For this review, take the finished solid that the model builds, in its own axes (mm). Face numbers are marked on the shaded views. A direction names the side the tool comes from. Give positions to 0.01 mm unless a question says otherwise; leave off trailing zeros. Loops run counter-clockwise (first coordinate to the right, second up) from the corner with the lowest first, then second, coordinate; pieces in that order, holes last. Notation, with made-up numbers: (-13, -10) - (13, -10) arc R11 ccw to (13, 1) - close; hole circle Ø7 at (27, 43.5). An arc over 180 degrees is marked (long way). Put each result on its own line as item: value. Start each with the question number.
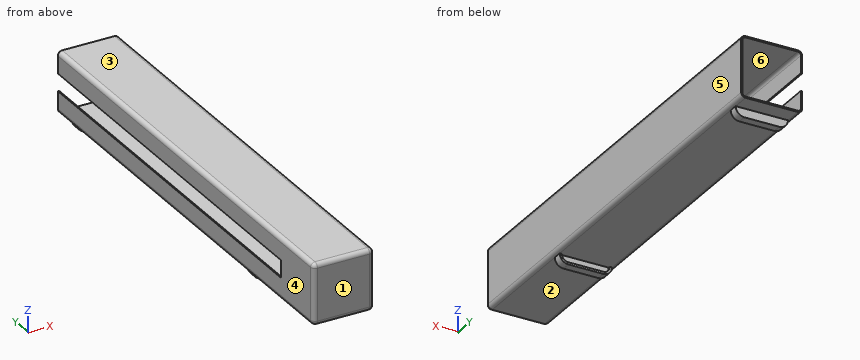
Autodesk Inventor part; units mm, degrees
ref_plane "YZ Plane" through (0, 0, 0) normal (1, 0, 0) x (0, 1, 0)
ref_plane "XY Plane" through (0, 0, 0) normal (0, 0, 1) x (1, 0, 0)
sketch "草图1" plane through (0, 0, 0) normal (0, 1, 0) x (-1, 0, 0)
  line L0 (0, 0) -> (-70, 0)
  line L1 (-70, 0) -> (-70, -70)
  line L2 (-70, -70) -> (0, -70)
  line L3 (0, -70) -> (0, 0)
  dimension "d0" = 70
  dimension "d1" = 70
extrude "拉伸1" add sketch "草图1" along normal blind 5
sketch "草图2" plane through (0, 5, 0) normal (0, 1, 0) x (1, 0, 0)
  line L0 (0, 70) -> (0, 0)
  line L1 (70, 70) -> (0, 70)
  line L2 (0, 0) -> (70, 0)
  line L3 (70, 0) -> (70, 70)
  line L4 (70, 70) -> (0, 70)
  line L5 (0, 70) -> (0, 0)
  line L6 (60, 60) -> (60, 10)
  line L7 (60, 10) -> (10, 10)
  line L8 (10, 10) -> (10, 60)
  line L9 (10, 60) -> (60, 60)
  dimension "d4" = 10
extrude "拉伸2" add sketch "草图2" along normal blind 60
fillet "圆角1" radius 5 8 edges at (0, 32.5, 0) (35, 0, 0) (0, 0, -35) (35, 0, -70) (70, 0, -35) (70, 32.5, -70) (70, 32.5, 0) (0, 32.5, -70)
sketch "草图3" plane through (0, 65, 0) normal (0, 1, 0) x (1, 0, 0)
  arc A0 (0, 5) -> (5, 0) centre (5, 5) ccw
  line L0 (5, 0) -> (65, 0)
  arc A1 (65, 0) -> (70, 5) centre (65, 5) ccw
  line L1 (70, 5) -> (70, 65)
  arc A2 (70, 65) -> (65, 70) centre (65, 65) ccw
  line L2 (65, 70) -> (5, 70)
  arc A3 (5, 70) -> (0, 65) centre (5, 65) ccw
  line L3 (0, 65) -> (0, 5)
  line L4 (60, 60) -> (60, 10)
  line L5 (60, 10) -> (10, 10)
  line L6 (10, 10) -> (10, 60)
  line L7 (10, 60) -> (60, 60)
  line L8 (68.5, 65) -> (68.5, 5)
  arc A4 (65, 1.5) -> (68.5, 5) centre (65, 5) ccw
  line L9 (65, 1.5) -> (5, 1.5)
  arc A5 (1.5, 5) -> (5, 1.5) centre (5, 5) ccw
  line L10 (1.5, 5) -> (1.5, 65)
  arc A6 (5, 68.5) -> (1.5, 65) centre (5, 65) ccw
  line L11 (5, 68.5) -> (65, 68.5)
  arc A7 (68.5, 65) -> (65, 68.5) centre (65, 65) ccw
  line L12 (1.5, 45) -> (0, 45)
  line L13 (0, 65) -> (0, 5)
  line L14 (1.5, 25) -> (0, 25)
  point P0 (0, 0)
  dimension "d8" = 1.5
  dimension "d9" = 25
  dimension "d10" = 25
extrude "拉伸3" add sketch "草图3" along normal blind 450 contours L3 L14 L10 A5 L9 A4 L8 A7 L11 A6 L12 A3 L2 A2 L1 A1 L0 A0
ref_plane "工作平面1" through (0, 130, 0) normal (0, 1, 0) x (-1, 0, 0)
sketch "草图5" plane through (0, 130, 0) normal (0, 1, 0) x (-1, 0, 0)
  arc A0 (-70, -65) -> (-65, -70) centre (-65, -65) ccw
  line L0 (-65, -70) -> (-5, -70)
  line L1 (-5, -70) -> (-5, -80)
  line L2 (-5, -80) -> (-65, -80)
  line L3 (-65, -80) -> (-65, -70)
  point P0 (0, 0)
  dimension "d18" = 10
extrude "拉伸4" add sketch "草图5" along normal blind 10
fillet "圆角2" radius 10 2 edges at (65, 135, -80) (5, 135, -80)
sketch "草图6" plane through (0, 140, 0) normal (0, 1, 0) x (1, 0, 0)
  point P0 (0, 0)
sketch "草图7" plane through (0, 140, 0) normal (0, 1, 0) x (1, 0, 0)
  arc A0 (65, 70) -> (55, 80) centre (55, 70) ccw
  line L0 (55, 80) -> (15, 80)
  arc A1 (15, 80) -> (5, 70) centre (15, 70) ccw
  arc A2 (62.5, 70) -> (55, 77.5) centre (55, 70) ccw
  line L1 (55, 77.5) -> (15, 77.5)
  arc A3 (15, 77.5) -> (7.5, 70) centre (15, 70) ccw
  line L2 (62.5, 70) -> (7.5, 70)
  line L3 (60, 10) -> (60, 60)
  point P0 (0, 0)
  dimension "d22" = 2.5
extrude "拉伸5" cut sketch "草图7" against normal blind 2
ref_plane "工作平面2" through (0, 485, 0) normal (0, 1, 0) x (1, 0, 0)
sketch "草图8" plane through (0, 485, 0) normal (0, 1, 0) x (1, 0, 0)
  arc A0 (15, 80) -> (5, 70) centre (15, 70) ccw
  line L0 (55, 80) -> (15, 80)
  arc A1 (65, 70) -> (55, 80) centre (55, 70) ccw
  line L1 (5, 70) -> (65, 70)
  point P0 (0, 0)
extrude "拉伸6" add sketch "草图8" along normal blind 10
sketch "草图9" plane through (0, 485, 0) normal (0, -1, 0) x (1, 0, 0)
  line L0 (15, -77.5) -> (55, -77.5)
  arc A0 (7.5, -70) -> (15, -77.5) centre (15, -70) ccw
  line L1 (62.5, -70) -> (7.5, -70)
  arc A1 (55, -77.5) -> (62.5, -70) centre (55, -70) ccw
  point P0 (0, 0)
extrude "拉伸7" cut sketch "草图9" against normal blind 2
properties part number "龙门架柱1"
1) Mouldability with a two-part tool opening along X and no side actions: class the marked faces 3, 4, 5 and 6 as released by +X, released by -X, zero draft, split by the parting line, or undercut.
2) Insertion check: P1, Ø2, axis at x = 31.5, z = -75, coming from the +Y side; P2, Ø10, axis at x = 35, y = 509, coming from the -Z side; P3, Ø8, axis at x = 36.5, z = -73, coming from the -Y side. Each pin has a flat end and moves straight along its axis. Give the tip position at first contact, or say it passes through.
3) Wall thickness on probe 1 along X at (y, z) = (208, -16); probe 2 along Z at (x, y) = (18.5, 410.5); probe 3 along Y at (x, z) = (42.5, -73): over which ranges is each line inside the solid? List them lowest first.
4) Take a section at A-A on x = 25.5. State the section outline as (y, z) points.
5) Take a section at B-B on y = 436.5. State the section outline as (x, z) points, and give its area (3 significant figures).
6) Machinability: for the marked faces 1 and 2, which of the approach directions +Z, -Z, +X, -X, +Y, -Y give a long, thin tool a straight path to every point of the face, cutting with its end or side? Answer none if there is none.
7) Take a section at C-C on z = -40.5. State the section outline as (x, y) points, and give its area (3 significant figures).
Answers follow:
1. face 3: zero draft
1. face 4: released by -X
1. face 5: released by +X
1. face 6: undercut
2. P1: y = 495
2. P2: z = -70
2. P3: y = 2
3. probe 1: 0 to 1.5, 68.5 to 70
3. probe 2: -70 to -68.5, -1.5 to 0
3. probe 3: 130 to 138, 487 to 495
4. outline: (0, -65) arc R5 ccw to (5, -70) - (130, -70) - (130, -80) - (140, -80) - (140, -77.5) - (138, -77.5) - (138, -70) - (487, -70) - (487, -77.5) - (485, -77.5) - (485, -80) - (495, -80) - (495, -70) - (515, -70) - (515, -68.5) - (65, -68.5) - (65, -60) - (5, -60) - (5, -10) - (65, -10) - (65, -1.5) - (515, -1.5) - (515, 0) - (5, 0) arc R5 ccw to (0, -5) - close
5. outline: (0, -65) arc R5 ccw to (5, -70) - (65, -70) arc R5 ccw to (70, -65) - (70, -5) arc R5 ccw to (65, 0) - (5, 0) arc R5 ccw to (0, -5) - (0, -25) - (1.5, -25) - (1.5, -5) arc R3.5 cw to (5, -1.5) - (65, -1.5) arc R3.5 cw to (68.5, -5) - (68.5, -65) arc R3.5 cw to (65, -68.5) - (5, -68.5) arc R3.5 cw to (1.5, -65) - (1.5, -45) - (0, -45) - close
5. area: 370 mm2
6. face 1: +Z, -Z, +X, -X, -Y
6. face 2: -Z, +X, -X, -Y
7. outline: (0, 5) arc R5 ccw to (5, 0) - (65, 0) arc R5 ccw to (70, 5) - (70, 515) - (68.5, 515) - (68.5, 65) - (60, 65) - (60, 5) - (10, 5) - (10, 65) - (0, 65) - close
7. area: 2,210 mm2
